For this review, take the finished solid that the model builds, in its own axes (mm). A direction names the side the tool comes from. Give positions to 0.01 mm unless a question says otherwise; leave off trailing zeros. Write each loop counter-clockwise with the first axis right and the second up, starting at its lowest first coordinate (ties: lowest second). Pieces come first, ordered by that corner, then holes.
Q1. Mouldability with a two-part tool opening along X and no side actions: class faces 1 (the cylindrical face through (8.255, -0.448, -0.017)), 2 (the flat face through (0, 3.175, 4)), 3 (the flat face through (-5.08, 0, -3)) as released by +X, released by -X, zero draft, split by the parting line, or undercut.
Q2. We need section D-D (x = -7.5). Write out the cut boundary in (y, z), then the cut area to 3 significant figures.
Q3. Insertion check: P1, Ø0.6, axis at x = 0, z = 3, coming from the +Y side (3 decimals); P2, Ø2, axis at x = 0, z = 9, coming from the +Y side; P3, Ø2.5, axis at x = -1, z = 4, coming from the -Y side (3 decimals); P4, Ø1.9, axis at x = -7.18, y = 0, coming from the -Z side. Each pin has a flat end and moves straight along its axis. Give the tip position at first contact, or say it passes through.
Q4. Machinability: for faces 4 (the flat face through (0, 3.175, -3)), 5 (the flat face through (5.08, 0, -3)), 6 (the cylindrical face through (3.916, -2.248, 8.307)), 7 (the flat face through (-3.329, 0.786, 3.623)), which of the approach directions +Z, -Z, +X, -X, +Y, -Y give a long, thin tool a straight path to every point of the face, cutting with its end or side? Answer none if there is none.
Q5. We need section C-C (z = 1.5). Write out the cut boundary in (x, y) (3 decimals), then the cut area to 3 significant figures.
Q6. For line 1 (Y direction, x = 0.75, z = 1.75) (3 decimals); line 2 (Z direction, x = 3.75, y = -2.75); line 3 (X direction, y = -1.5, z = 6.75), list the stretches that pass through material, from the lowest coordinate up.
Q7. We need section A-A (y = 0). Write out the cut boundary in (x, z).
Q8. We need section B-B (x = 6.25). Write out the cut boundary in (y, z), then the cut area to 3 significant figures.
```python
from build123d import *

# Parameters (mm, degrees)
F0_R     = 1.1684
F1_DEPTH = 1.1811
F3_DEPTH = 4.953
F5_DEPTH = 3.5814
F7_DEPTH = 4.4069


with BuildPart() as f1:
    # F0 (on Top) → F1 (new body, symmetric)
    with BuildSketch(Plane.XY):
        with BuildLine():
            Line((8.3947, 3.9116), (-8.3947, 3.9116))
            ThreePointArc((-8.3947, 3.9116), (-9.508252, 3.450352), (-9.9695, 2.3368))
            Line((-9.9695, 2.3368), (-9.9695, -2.3368))
            ThreePointArc((-9.9695, -2.3368), (-9.508252, -3.450352), (-8.3947, -3.9116))
            Line((-8.3947, -3.9116), (8.3947, -3.9116))
            ThreePointArc((8.3947, -3.9116), (9.508252, -3.450352), (9.9695, -2.3368))
            Line((9.9695, -2.3368), (9.9695, 2.3368))
            ThreePointArc((9.9695, 2.3368), (9.508252, 3.450352), (8.3947, 3.9116))
        make_face()
        with Locations((-7.1755, 0)):
            Circle(F0_R, mode=Mode.SUBTRACT)
        with Locations((7.1755, 0)):
            Circle(F0_R, mode=Mode.SUBTRACT)
    extrude(amount=F1_DEPTH, both=True)

    # F2 (on face) → F3 (join)
    with BuildSketch(Plane.XY.offset(1.1811)):
        with BuildLine():
            Line((-2.85102, -3.175), (2.852478, -3.175))
            ThreePointArc((2.852478, -3.175), (4.209371, -2.399471), (4.229829, -0.836722))
            Line((4.229829, -0.836722), (2.455818, 2.363678))
            ThreePointArc((2.455818, 2.363678), (1.877738, 2.957094), (1.078467, 3.175))
            Line((1.078467, 3.175), (-1.077009, 3.175))
            ThreePointArc((-1.077009, 3.175), (-1.876281, 2.957094), (-2.454361, 2.363678))
            Line((-2.454361, 2.363678), (-4.228371, -0.836722))
            ThreePointArc((-4.228371, -0.836722), (-4.207914, -2.399471), (-2.85102, -3.175))
        make_face()
    extrude(amount=F3_DEPTH)

    # F4 (on face) → F5 (join)
    with BuildSketch(Plane(origin=(0, 0, -1.1811), x_dir=(1, 0, 0), z_dir=(0, 0, -1))):
        with BuildLine():
            Line((3.5052, 3.175), (-3.5052, 3.175))
            ThreePointArc((-3.5052, 3.175), (-4.618752, 2.713752), (-5.08, 1.6002))
            Line((-5.08, 1.6002), (-5.08, -1.6002))
            ThreePointArc((-5.08, -1.6002), (-4.618752, -2.713752), (-3.5052, -3.175))
            Line((-3.5052, -3.175), (3.5052, -3.175))
            ThreePointArc((3.5052, -3.175), (4.618752, -2.713752), (5.08, -1.6002))
            Line((5.08, -1.6002), (5.08, 1.6002))
            ThreePointArc((5.08, 1.6002), (4.618752, 2.713752), (3.5052, 3.175))
        make_face()
    extrude(amount=F5_DEPTH)

    # F6 (on face) → F7 (join)
    with BuildSketch(Plane.XY.offset(6.1341)):
        with BuildLine():
            Line((0.891445, 2.8575), (-0.889988, 2.8575))
            ThreePointArc((-0.889988, 2.8575), (-1.689259, 2.639594), (-2.267339, 2.046178))
            Line((-2.267339, 2.046178), (-3.940227, -0.971792))
            ThreePointArc((-3.940227, -0.971792), (-3.923729, -2.232074), (-2.82946, -2.8575))
            Line((-2.82946, -2.8575), (2.830917, -2.8575))
            ThreePointArc((2.830917, -2.8575), (3.925186, -2.232074), (3.941684, -0.971792))
            Line((3.941684, -0.971792), (2.268796, 2.046178))
            ThreePointArc((2.268796, 2.046178), (1.690717, 2.639594), (0.891445, 2.8575))
        make_face()
    extrude(amount=F7_DEPTH)


solid = f1.part
```
Computed:
1. face 1: undercut
1. face 2: zero draft
1. face 3: released by -X
2. outline: (-3.91, -1.18) - (-1.12, -1.18) - (-1.12, 1.18) - (-3.91, 1.18) - close; (1.12, -1.18) - (3.91, -1.18) - (3.91, 1.18) - (1.12, 1.18) - close
2. area: 13.2 mm2
3. P1: stops at y = 3.175
3. P2: stops at y = 2.86
3. P3: stops at y = -3.175
3. P4: passes through
4. face 4: -Z, +X, -X, +Y
4. face 5: -Z, +X, +Y, -Y
4. face 6: +Z, +X
4. face 7: +Z, -X, +Y
5. outline: (-4.228, -0.837) arc R1.575 ccw to (-2.851, -3.175) - (2.852, -3.175) arc R1.575 ccw to (4.23, -0.837) - (2.456, 2.364) arc R1.575 ccw to (1.078, 3.175) - (-1.077, 3.175) arc R1.575 ccw to (-2.454, 2.364) - close
5. area: 44.3 mm2
6. line 1: y = -3.175 to 3.175
6. line 2: z = -4.76 to 6.13
6. line 3: x = -4.1 to 4.1
7. outline: (-9.97, -1.18) - (-8.34, -1.18) - (-8.34, 1.18) - (-9.97, 1.18) - close; (-6.01, -1.18) - (-5.08, -1.18) - (-5.08, -4.76) - (5.08, -4.76) - (5.08, -1.18) - (6.01, -1.18) - (6.01, 1.18) - (3.77, 1.18) - (3.77, 6.13) - (3.4, 6.13) - (3.4, 10.54) - (-3.4, 10.54) - (-3.4, 6.13) - (-3.76, 6.13) - (-3.76, 1.18) - (-6.01, 1.18) - close; (8.34, -1.18) - (9.97, -1.18) - (9.97, 1.18) - (8.34, 1.18) - close
8. outline: (-3.91, -1.18) - (-0.71, -1.18) - (-0.71, 1.18) - (-3.91, 1.18) - close; (0.71, -1.18) - (3.91, -1.18) - (3.91, 1.18) - (0.71, 1.18) - close
8. area: 15.1 mm2
